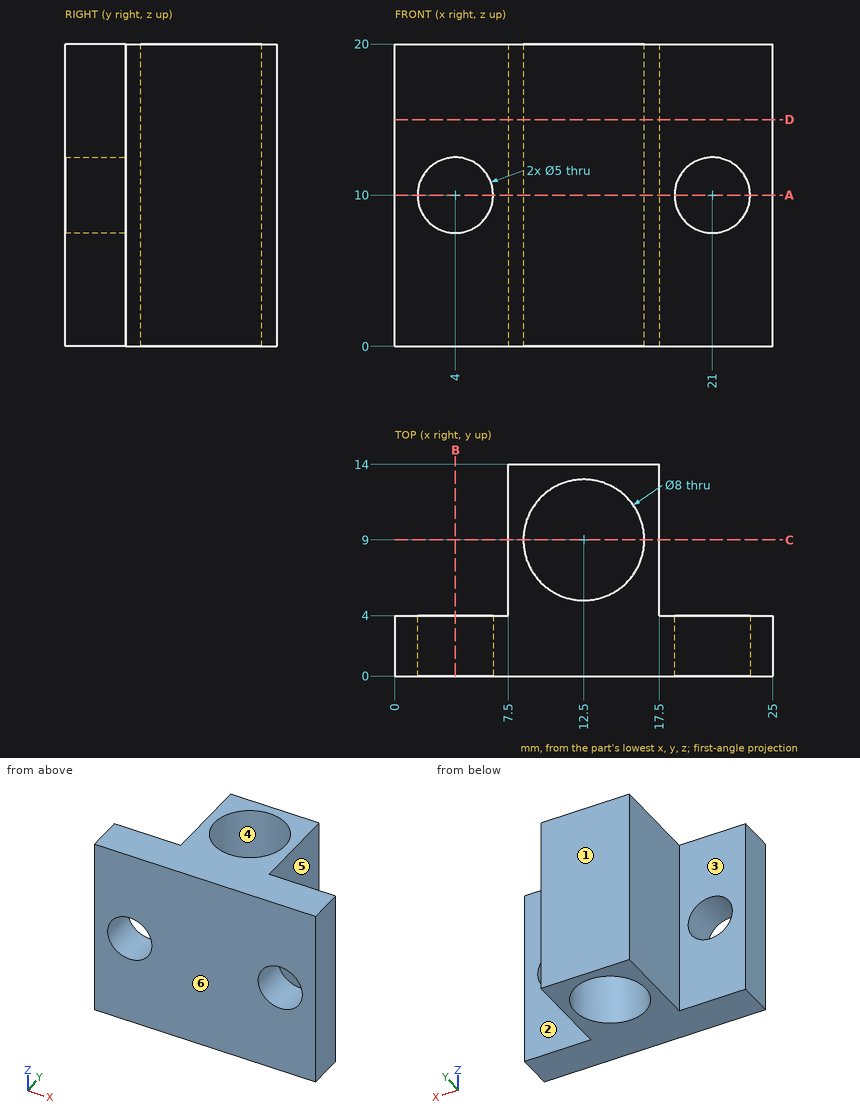
Study the drawing (mm; zero at the part's minimum x, y, z) and answer. A direction names the side the tool comes from. Give positions to 0.01 mm unless a question says otherwise; leave off trailing zeros. Write each loop counter-clockwise with the first axis right and the second up, starting at its lowest first coordinate (ties: lowest second). Pieces come first, ordered by that corner, then holes. Notation, with made-up numbers: (86.5, 2) -> (100.5, 2) arc R12 ccw to (100.5, 22) -> close; hole circle Ø9 at (34.5, -10.75). An arc over 180 degrees is marked (long way). Answer as a JSON object with one key per item and string values. Group by question number.
1) Consider L1, parallel to X at y = 9, z = 7.75; L2, parallel to Y at x = 12.5, z = 8.75; L3, parallel to X at y = 7.5, z = 10.5. Determine where each line is inside the solid, lowest interval first. Write a range as from..to.
2) Each of these flat-tipped pins is pushed along its axis until it touches: P1, Ø8, axis at y = 11, z = 8.5, coming from the +X side; P2, Ø1, axis at y = 12, z = 9.5, coming from the -X side; P3, Ø4, axis at x = 4, z = 10, coming from the +Y side; P4, Ø8, axis at x = 3, z = 6, coming from the +Y side. Where does it stop, or does it pass through?
3) Find section A-A (z = 10). Write down the section's boundary in (x, y).
4) Find section B-B (x = 4). Write down the section's boundary in (y, z), and give its area (3 significant figures).
5) A tool of negligible diameter and unlimited length cuts with its end or side. For the marked faces 1, 2 and 3, from which of +Z, -Z, +X, -X, +Y, -Y can it reach the whole face along a straight path? Write none if from no direction.
6) The mould has two halves that part along Y. Classify the marked faces 4, 5 and 6: +Y half, -Y half, draft (parallel to the pull), parting line (faces both ways), or undercut.
7) Find section C-C (y = 9). Write down the section's boundary in (x, z), and give its area (3 significant figures).
8) Find section D-D (z = 15). Write down the section's boundary in (x, y), and give its area (3 significant figures).
Values follow:
{
 "1": {"L1": "x = 7.5..8.5, 16.5..17.5", "L2": "y = 0..5, 13..14", "L3": "x = 7.5..8.79, 16.21..17.5"},
 "2": {"P1": "stops at x = 17.5", "P2": "stops at x = 7.5", "P3": "passes through", "P4": "stops at y = 4"},
 "3": {"outline": "(0, 0) -> (1.5, 0) -> (1.5, 4) -> (0, 4) -> close; (6.5, 0) -> (18.5, 0) -> (18.5, 4) -> (17.5, 4) -> (17.5, 14) -> (7.5, 14) -> (7.5, 4) -> (6.5, 4) -> close; (23.5, 0) -> (25, 0) -> (25, 4) -> (23.5, 4) -> close; hole circle Ø8 at (12.5, 9)"},
 "4": {"outline": "(0, 0) -> (4, 0) -> (4, 7.5) -> (0, 7.5) -> close; (0, 12.5) -> (4, 12.5) -> (4, 20) -> (0, 20) -> close", "area": "60.0 mm2"},
 "5": {"face 1": "+Z, -Z, +X, -X, +Y", "face 2": "+Z, -Z, +X, +Y", "face 3": "+Z, -Z, -X, +Y"},
 "6": {"face 4": "undercut", "face 5": "draft", "face 6": "-Y half"},
 "7": {"outline": "(7.5, 0) -> (8.5, 0) -> (8.5, 20) -> (7.5, 20) -> close; (16.5, 0) -> (17.5, 0) -> (17.5, 20) -> (16.5, 20) -> close", "area": "40.0 mm2"},
 "8": {"outline": "(0, 0) -> (25, 0) -> (25, 4) -> (17.5, 4) -> (17.5, 14) -> (7.5, 14) -> (7.5, 4) -> (0, 4) -> close; hole circle Ø8 at (12.5, 9)", "area": "150 mm2"}
}
